Study the drawing (mm; zero at the part's minimum x, y, z) and answer. A direction names the side the tool comes from. Coordinates: 2 decimals unless noted, no trailing zeros. Loops run counter-clockwise (first coordinate to the right, second up) from the corner with the lowest first, then second, coordinate; pieces in that order, holes last. Notation, with made-up numbers: (45, -0.5) - (78, -0.5) arc R20 ccw to (78, 4.5) - close; hole circle Ø4 at (39, 17). An arc over 180 degrees is marked (long way). Use CSV: the item, a comma, the result in double quotes.
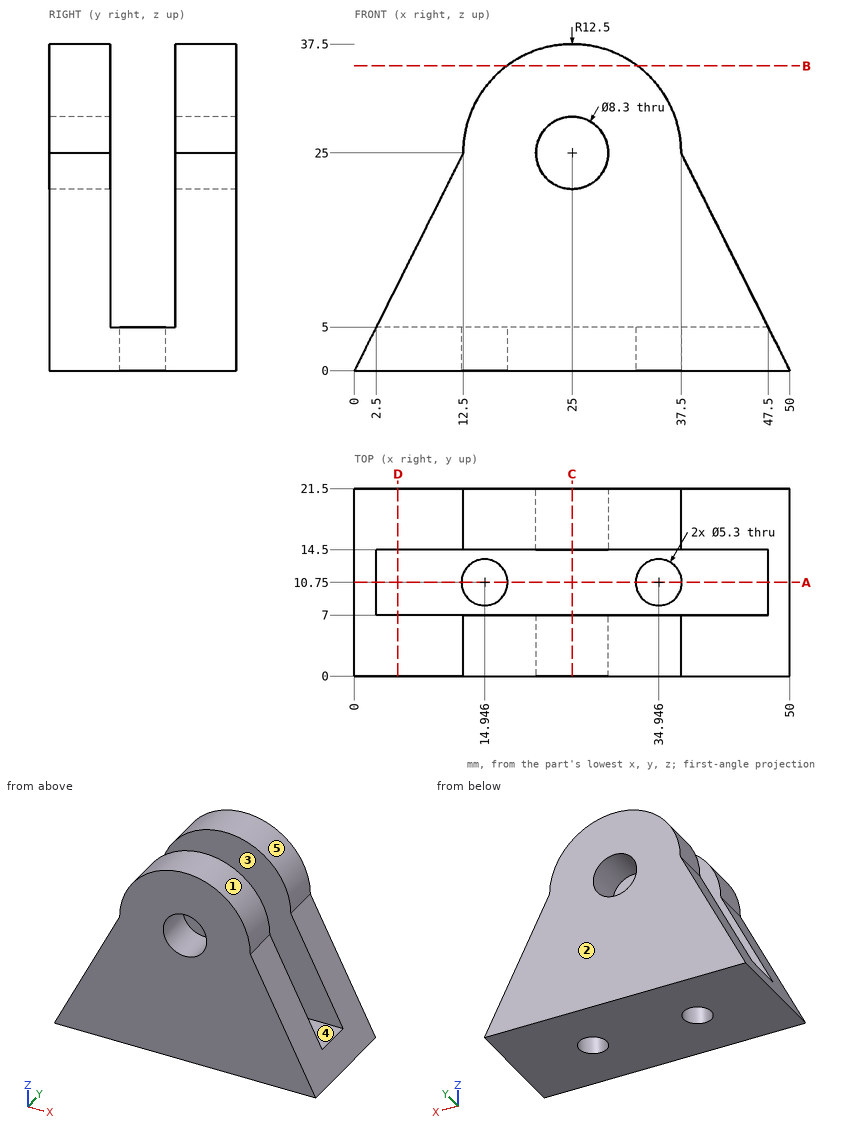
Q1. The part is cut by section A-A on y = 10.75. Determine the outline of the cut face in (x, z) (1 decimal).
Reported:
outline,"(0, 0) - (12.3, 0) - (12.3, 5) - (2.5, 5) - close; (17.6, 0) - (32.3, 0) - (32.3, 5) - (17.6, 5) - close; (37.6, 0) - (50, 0) - (47.5, 5) - (37.6, 5) - close"
Q2. A tool of negligible diameter and unlimited length cuts with its end or side. For the marked faces 4 and 5, from which of +Z, -Z, +X, -X, +Y, -Y can it reach the whole face along a straight path? Write none if from no direction.
Reported:
face 4,"+Z, +X, -X"
face 5,"+Z, +Y, -Y"
Q3. The part is cut by section C-C on x = 25. Determine the outline of the cut face in (y, z), and give its area (3 significant figures).
Reported:
outline,"(0, 0) - (21.5, 0) - (21.5, 20.85) - (14.5, 20.85) - (14.5, 5) - (7, 5) - (7, 20.85) - (0, 20.85) - close; (0, 29.15) - (7, 29.15) - (7, 37.5) - (0, 37.5) - close; (14.5, 29.15) - (21.5, 29.15) - (21.5, 37.5) - (14.5, 37.5) - close"
area,"446 mm²"
Q4. The part is cut by section B-B on z = 35. Determine the outline of the cut face in (x, y), and give its area (3 significant figures).
Reported:
outline,"(17.5, 0) - (32.5, 0) - (32.5, 7) - (17.5, 7) - close; (17.5, 14.5) - (32.5, 14.5) - (32.5, 21.5) - (17.5, 21.5) - close"
area,"210 mm²"
Q5. Find the intervals of material crossed by probe 1 along X at (y, z) = (16, 25); probe 2 along Y at (x, z) = (19.5, 25.5); probe 3 along Y at (x, z) = (15, 4), in increasing order. Write a range as [from, to].
Reported:
probe 1,"x = [12.5, 20.85], [29.15, 37.5]"
probe 2,"y = [0, 7], [14.5, 21.5]"
probe 3,"y = [0, 8.1], [13.4, 21.5]"
Q6. The part is cut by section D-D on x = 5. Determine the outline of the cut face in (y, z).
Reported:
outline,"(0, 0) - (21.5, 0) - (21.5, 10) - (14.5, 10) - (14.5, 5) - (7, 5) - (7, 10) - (0, 10) - close"
Q7. Given P1, Ø2, axis at x = 7.5, y = 11.5, coming from the +Z side; P2, Ø8.5, axis at x = 34.95, y = 10.75, coming from the +Z side (1 decimal); P3, Ø12, axis at y = 15, z = 18.5, coming from the -X side; P4, Ø3, axis at x = 14.95, y = 10.75, coming from the +Z side, each flat-ended and moving along its own axis, determine where each tip first touches the part or whether it passes through.
Reported:
P1,"stops at z = 5"
P2,"stops at z = 34.6"
P3,"stops at x = 6.25"
P4,"passes through"
Q8. For a pull along Y with two mould halves and no side action, classify the marked faces 1, 2 and 3 as +Y half, -Y half, draft (parallel to the pull), parting line (faces both ways), or undercut.
Reported:
face 1,"draft"
face 2,"+Y half"
face 3,"undercut"
